The listing builds one solid part. Answer for the finished solid, in the listing's coordinates (mm). A direction names the side the tool comes from. Round coordinates to 2 decimals unless told otherwise and drop trailing zeros. Write each loop counter-clockwise with the first axis right and the second up, starting at its lowest first coordinate (ties: lowest second). Pieces come first, ordered by that corner, then holes. Notation, with made-up numbers: M 53.5,-40 L 106.5,-40 A26 ccw 106.5,-2 Z; hole C 34.25,-37.5 d9. An arc over 180 degrees is marked long. One line per item, written item: value. Start each with the question number.
(1) Consider probe 1 along X at (y, z) = (28, 2.7); probe 2 along Y at (x, z) = (-25, 7); probe 3 along Y at (x, z) = (25, 1). Determine where each line is inside the solid, lowest interval first.
(2) Section A-A (y = 28) is taken. Determine the outline of the cut face in (x, z).
(3) Section C-C (x = 8.5) is taken. Determine the outline of the cut face in (y, z).
(4) Section B-B (z = -55.5) is taken. Determine the outline of the cut face in (x, y).
(5) For faces 4 (the flat face through (3, 19, -34)), 5 (the flat face through (19.5, 13, -37)), 6 (the cylindrical face through (-24.284, 33.453, 2.958)), 7 (the flat face through (0, -6, 4)), determine the directions among +Z, -Z, +X, -X, +Y, -Y from which every point of the face is accessible in a straight line to the end or side of a thin tool.
(6) Section D-D (y = 14) is taken. Determine the outline of the cut face in (x, z), plus the area to 3 significant figures.
(7) Given P1, Ø5.5, axis at x = 27, y = -22, coming from the -Z side; P2, Ø8, axis at x = 25, y = 28, coming from the +Z side; P3, Ø3, axis at x = -16, z = -37, coming from the +Y side; P4, Ø4, axis at x = 11.5, z = -34.5, coming from the -Y side, each flat-ended and moving along its own axis, determine where each tip first touches the part or whether it passes through.
(8) For a pull along Y with two mould halves and no side action, classify faces 1 (the flat face through (0, 39, 4)), 2 (the flat face through (25, 24, 6)), 3 (the flat face through (34, 10, -21)) as released by +Y, released by -Y, zero draft, split by the parting line, or undercut.
```python
from build123d import *

# Parameters (mm, degrees)
SKETCH1_W           = 68
SKETCH1_H           = 78
BOSS_EXTRUDE1_DEPTH = 8
BOSS_EXTRUDE2_DEPTH = 75
CUT_EXTRUDE1_REACH  = 85
SKETCH3_W           = 43
SKETCH3_H           = 15
FILLET1_R           = 2
FILLET2_R           = 5
SKETCH4_W           = 6
SKETCH4_H           = 45
CUT_EXTRUDE2_DEPTH  = 62.5
SKETCH5_R           = 3.5
CUT_EXTRUDE3_DEPTH  = 9
SKETCH7_R           = 5.5
CUT_EXTRUDE4_DEPTH  = 6


with BuildPart() as part:
    # Sketch1 → Boss-Extrude1 (new body)
    with BuildSketch(Plane.XY):
        Rectangle(SKETCH1_W, SKETCH1_H)
    extrude(amount=BOSS_EXTRUDE1_DEPTH)

    # Sketch2 → Boss-Extrude2 (add)
    with BuildSketch(Plane(origin=(0, 0, 0), x_dir=(-1, 0, 0), z_dir=(0, 0, -1))):
        Polygon((-34, 22.5), (34, 22.5), (34, 9.5), (19.5, 9.5), (19.5, 15.5), (-19.5, 15.5), (-19.5, 9.5), (-34, 9.5), align=None)
    extrude(amount=BOSS_EXTRUDE2_DEPTH)

    # Sketch3 → Cut-Extrude1 (cut, up to next)
    with BuildSketch(Plane.XY.offset(8), mode=Mode.PRIVATE) as cut_extrude1_sk1:
        with Locations((0, 1.5)):
            Rectangle(SKETCH3_W, SKETCH3_H)
    cut_extrude1_tool1 = extrude(cut_extrude1_sk1.sketch, amount=-CUT_EXTRUDE1_REACH, mode=Mode.PRIVATE) & part.part
    add(cut_extrude1_tool1.solids().sort_by_distance((0, 1.5, 8))[0], mode=Mode.SUBTRACT)

    # Fillet1
    fillet1_edges = [part.edges().sort_by_distance(p)[0] for p in [
        (34, 16, -75),
        (-34, 16, -75),
        (-21.5, -6, 4),
        (-21.5, 9, 4),
        (21.5, 9, 4),
        (21.5, -6, 4),
    ]]
    fillet(fillet1_edges, radius=FILLET1_R)

    # Fillet2
    fillet2_edges = [part.edges().sort_by_distance(p)[0] for p in [
        (34, -39, 4),
        (-34, -39, 4),
        (-34, 39, 4),
        (34, 39, 4),
    ]]
    fillet(fillet2_edges, radius=FILLET2_R)

    # Sketch4 → Cut-Extrude2 (cut, through all)
    with BuildSketch(Plane(origin=(0, 22.5, 0), x_dir=(1, 0, 0), z_dir=(0, 1, 0))):
        with Locations((0, 34.5)):
            Rectangle(SKETCH4_W, SKETCH4_H)
    extrude(amount=-CUT_EXTRUDE2_DEPTH, mode=Mode.SUBTRACT)

    # Sketch5 → Cut-Extrude3 (cut, through all)
    with BuildSketch(Plane(origin=(0, 0, 0), x_dir=(-1, 0, 0), z_dir=(0, 0, -1))):
        with Locations((-25, 28)):
            Circle(SKETCH5_R)
        with Locations((25, 28)):
            Circle(SKETCH5_R)
        with Locations((-25, -22)):
            Circle(SKETCH5_R)
        with Locations((25, -22)):
            Circle(SKETCH5_R)
    extrude(amount=-CUT_EXTRUDE3_DEPTH, mode=Mode.SUBTRACT)

    # Sketch7 → Cut-Extrude4 (cut)
    with BuildSketch(Plane(origin=(0, 0, 0), x_dir=(-1, 0, 0), z_dir=(0, 0, -1))):
        with Locations((-25, 28)):
            Circle(SKETCH7_R)
        with Locations((25, 28)):
            Circle(SKETCH7_R)
        with Locations((-25, -22)):
            Circle(SKETCH7_R)
        with Locations((25, -22)):
            Circle(SKETCH7_R)
    extrude(amount=-CUT_EXTRUDE4_DEPTH, mode=Mode.SUBTRACT)


solid = part.part
```
Recorded:
1. probe 1: x = -34 to -30.5, -19.5 to 19.5, 30.5 to 34
1. probe 2: y = -39 to -25.5, -18.5 to 24.5, 31.5 to 39
1. probe 3: y = -39 to -27.5, -16.5 to 22.5, 33.5 to 39
2. outline: M -34,0 L -30.5,0 L -30.5,6 L -28.5,6 L -28.5,8 L -34,8 Z; M -21.5,6 L -19.5,6 L -19.5,0 L 19.5,0 L 19.5,6 L 21.5,6 L 21.5,8 L -21.5,8 Z; M 28.5,6 L 30.5,6 L 30.5,0 L 34,0 L 34,8 L 28.5,8 Z
3. outline: M -39,0 L -6,0 L -6,8 L -39,8 Z; M 9,0 L 15.5,0 L 15.5,-75 L 22.5,-75 L 22.5,0 L 39,0 L 39,8 L 9,8 Z
4. outline: M -34,9.5 L -19.5,9.5 L -19.5,15.5 L -3,15.5 L -3,22.5 L -34,22.5 Z; M 3,15.5 L 19.5,15.5 L 19.5,9.5 L 34,9.5 L 34,22.5 L 3,22.5 Z
5. face 4: +Y, -Y
5. face 5: -Z, -Y
5. face 6: -Z
5. face 7: +Z, -Z
6. outline: M -34,-73 A2 ccw -32,-75 L -19.5,-75 L -19.5,0 L 19.5,0 L 19.5,-75 L 32,-75 A2 ccw 34,-73 L 34,8 L -34,8 Z
6. area: 2,720 mm2
7. P1: stops at z = 6
7. P2: stops at z = 8
7. P3: stops at y = 22.5
7. P4: stops at y = 15.5
8. face 1: released by +Y
8. face 2: undercut
8. face 3: zero draft
